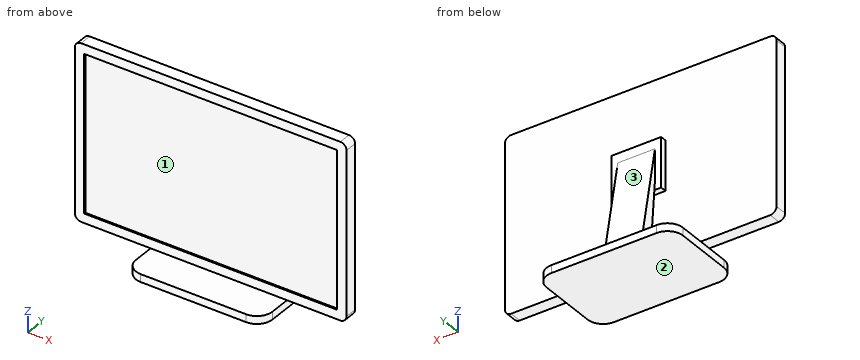
from build123d import *

# Parameters (mm, degrees)
F0_W      = 518.439682
F0_H      = 320.675
F1_DEPTH  = 25.4
F2_DEPTH  = 22.225
F3_W      = 101.6
F3_H      = 101.6
F4_DEPTH  = 12.7
F6_DEPTH  = 38.1
F7_W      = 184.15
F7_H      = 15.875
F8_DEPTH  = 101.6
F9_W      = 184.15
F9_H      = 15.875
F10_DEPTH = 101.6
F11_R     = 31.75


with BuildPart() as f1:
    # F0 (on Front) → F1 (new body)
    with BuildSketch(Plane.XZ):
        with BuildLine():
            Line((278.269841, -166.6875), (278.269841, 166.6875))
            ThreePointArc((278.269841, 166.6875), (274.550097, 175.667756), (265.569841, 179.3875))
            Line((265.569841, 179.3875), (-265.569841, 179.3875))
            ThreePointArc((-265.569841, 179.3875), (-274.550097, 175.667756), (-278.269841, 166.6875))
            Line((-278.269841, 166.6875), (-278.269841, -166.6875))
            ThreePointArc((-278.269841, -166.6875), (-274.550097, -175.667756), (-265.569841, -179.3875))
            Line((-265.569841, -179.3875), (265.569841, -179.3875))
            ThreePointArc((265.569841, -179.3875), (274.550097, -175.667756), (278.269841, -166.6875))
        make_face()
        Rectangle(F0_W, F0_H, mode=Mode.SUBTRACT)
    extrude(amount=F1_DEPTH)

    # F0 (on Front) → F2 (join)
    with BuildSketch(Plane.XZ):
        Rectangle(F0_W, F0_H)
    extrude(amount=F2_DEPTH)

    # F3 (on face) → F4 (join)
    with BuildSketch(Plane.XZ):
        Rectangle(F3_W, F3_H)
    extrude(amount=-F4_DEPTH)

    # F5 (on Right) → F6 (join, symmetric)
    with BuildSketch(Plane.YZ):
        Polygon((12.7, 31.75), (12.7, -31.75), (27.283267, -198.4375), (-76.2, -198.4375), (-76.2, -214.3125), (107.95, -214.3125), (107.95, -198.4375), (57.15, -198.4375), align=None)
    extrude(amount=F6_DEPTH, both=True)

    # F7 (on face) → F8 (join)
    with BuildSketch(Plane.YZ.offset(38.1)):
        with Locations((15.875, -206.375)):
            Rectangle(F7_W, F7_H)
    extrude(amount=F8_DEPTH)

    # F9 (on face) → F10 (join)
    with BuildSketch(Plane(origin=(-38.1, 0, 0), x_dir=(0, -1, 0), z_dir=(-1, 0, 0))):
        with Locations((-15.875, -206.375)):
            Rectangle(F9_W, F9_H)
    extrude(amount=F10_DEPTH)

    # F11
    f11_edges = [f1.edges().sort_by_distance(p)[0] for p in [
        (-139.7, 107.95, -206.375),
        (139.7, 107.95, -206.375),
        (139.7, -76.2, -206.375),
        (-139.7, -76.2, -206.375),
    ]]
    fillet(f11_edges, radius=F11_R)


solid = f1.part
The model under review builds one solid part; all positions refer to its coordinate system, in mm. Face numbers are marked on the shaded views. Round coordinates to 2 decimals unless told otherwise and drop trailing zeros. Order: outer loops, then holes, each group sorted by start corner. A loop starts at its lowest first (then second) coordinate and runs counter-clockwise, first axis right, second up. Notation, with made-up numbers: (-11, 44.25) - (46, 44.25) arc R33 cw to (46, 81.25) - close; hole circle Ø6 at (-4.5, 70). An arc over 180 degrees is marked (long way). Use one line per item in the form item = value.
Q1. Mouldability with a two-part tool opening along Z and no side actions: class the marked faces 1, 2 and 3 as pulls with the +Z half, pulls with the -Z half, needs draft (parallel to the pull), parting line crosses it, or undercut.
Response values:
face_1 = undercut
face_2 = pulls with the -Z half
face_3 = pulls with the +Z half
Q2. Add section C-C on z = 138.5. Give the boundary of the cut face in (x, y) (3 decimals), then the cut area to 3 significant figures.
Response values:
outline = (-278.27, -25.4) - (-259.22, -25.4) - (-259.22, -22.225) - (259.22, -22.225) - (259.22, -25.4) - (278.27, -25.4) - (278.27, 0) - (-278.27, 0) - close
area = 12,500 mm^2
Q3. To check wall thickness, follow line 1 (X direction, y = -23, z = -158.5); line 2 (Z direction, x = -123, y = -22); line 3 (Z direction, x = -217, y = -22.5). State the ranges of each line that lie inside material, in increasing order.
Response values:
line_1 = -278.27 to -259.22, 259.22 to 278.27
line_2 = -214.31 to -198.44, -179.39 to 179.39
line_3 = -179.39 to -160.34, 160.34 to 179.39
Q4. Add section B-B on z = -87. Give the boundary of the cut face in (x, y) (3 decimals).
Response values:
outline = (-278.27, -25.4) - (-259.22, -25.4) - (-259.22, -22.225) - (259.22, -22.225) - (259.22, -25.4) - (278.27, -25.4) - (278.27, 0) - (-278.27, 0) - close; (-38.1, 17.534) - (38.1, 17.534) - (38.1, 35.631) - (-38.1, 35.631) - close
Q5. Clearance check with flat-ended pins moving along their axes: P1, Ø3, axis at x = -19, y = -54, coming from the +Z side; P2, Ø17.5, axis at y = -9.5, z = -209.5, coming from the +X side; P3, Ø6, axis at x = -138, z = -39.5, coming from the -Y side (3 decimals); P4, Ø1.5, axis at y = 1.5, z = -105, coming from the +X side. State where each tip first meets the part, or that it passes through.
Response values:
P1 = -198.44
P2 = 139.7
P3 = -22.225
P4 = through
